```python
from build123d import *

# Parameters (mm, degrees)
F0_R     = 37.5
F1_DEPTH = 4
F2_R     = 37.5
F2_R_2   = 33.5
F3_DEPTH = 5
F4_R     = 35.6
F5_DEPTH = 5
F6_R     = 2.5
F7_DEPTH = 4.001
F8_R     = 5


with BuildPart() as f1:
    # F0 (on Top) → F1 (new body)
    with BuildSketch(Plane.XY):
        Circle(F0_R)
    extrude(amount=F1_DEPTH)

    # F2 (on face) → F3 (join)
    with BuildSketch(Plane.XY.offset(4)):
        Circle(F2_R)
        Circle(F2_R_2, mode=Mode.SUBTRACT)
    extrude(amount=F3_DEPTH)

    # F4 (on face) → F5 (cut)
    with BuildSketch(Plane.XY.offset(9)):
        Circle(F4_R)
    extrude(amount=-F5_DEPTH, mode=Mode.SUBTRACT)

    # F6 (on face) → F7 (cut, through all)
    with BuildSketch(Plane.XY.offset(4)):
        Circle(F6_R)
    extrude(amount=-F7_DEPTH, mode=Mode.SUBTRACT)

    # F8
    f8_edges = [f1.edges().sort_by_distance(p)[0] for p in [
        (-37.5, 0, 0),
    ]]
    fillet(f8_edges, radius=F8_R)


solid = f1.part
```
CAD build for the part. Positions are in the model's coordinates, mm. A direction names the side the tool comes from. Give positions to 0.01 mm unless a question says otherwise; leave off trailing zeros. Write each loop counter-clockwise with the first axis right and the second up, starting at its lowest first coordinate (ties: lowest second). Pieces come first, ordered by that corner, then holes. Notation, with made-up numbers: M 16,72 L 62,72 A18 cw 62,94 Z; hole C 37,16 d2. An arc over 180 degrees is marked long. Return JSON: item names as keys, results as strings. Group by question number.
(1) Flat gauge pins, fed straight in: pin 1 Ø5 at (x, y) = (15.5, -18.5) entering from +Z; pin 2 Ø6.5 at (x, y) = (0, 0) entering from -Z; pin 3 Ø3 at (x, z) = (-6, 5) entering from -Y; pin 4 Ø2 at (x, z) = (-5.5, 7) entering from +Y. Where does each tip first touch, or does it go through?
(2) Drill centre lines: L1, parallel to Y at x = 0, z = 7.7; L2, parallel to Z at x = 3.5, y = -16.5; L3, parallel to Y at x = 0, z = 2.5. Where is each one in solid material? Low to high. Write a range as [from, to].
(3) Band-saw the part on A-A (y = 0). Give the cut face in (x, z).
(4) 3-axis set-ups, long thin cutter, end or side, ignore diameter. For faces 4 (the face through (33, -14, 9)), 5 (the face through (0, -7, 4)): which of +Z, -Z, +X, -X, +Y, -Y reach the whole face in a straight line?
(5) Mould opens along X. For faces 1 (the face through (-4.88, 37.18, 6.97)), 2 (the face through (7, 0, 0)), 3 (the face through (-0.54, -2.44, 2.03)) say: pulls with the +X half, pulls with the -X half, needs draft (parallel to the pull), parting line crosses it, or undercut.
(6) Band-saw the part on C-C (z = 6.25). Give the cut face in (x, y), and give its area (3 significant figures).
(7) Band-saw the part on D-D (z = 1). Give the cut face in (x, y), and give its area (3 significant figures).
Entries:
{
 "1": {"pin 1": "stops at z = 4", "pin 2": "stops at z = 0", "pin 3": "stops at y = -37.23", "pin 4": "stops at y = 37.23"},
 "2": {"L1": "y = [-37.5, -35.6], [35.6, 37.5]", "L2": "z = [0, 4]", "L3": "y = [-36.83, -2.5], [2.5, 36.83]"},
 "3": {"outline": "M -37.5,5 A5 ccw -32.5,0 L -2.5,0 L -2.5,4 L -35.6,4 L -35.6,9 L -37.5,9 Z; M 2.5,0 L 32.5,0 A5 ccw 37.5,5 L 37.5,9 L 35.6,9 L 35.6,4 L 2.5,4 Z"},
 "4": {"face 4": "+Z, +X, -X, +Y, -Y", "face 5": "+Z"},
 "5": {"face 1": "parting line crosses it", "face 2": "needs draft", "face 3": "undercut"},
 "6": {"outline": "C 0,0 d75; hole C 0,0 d71.2", "area": "436 mm^2"},
 "7": {"outline": "C 0,0 d71; hole C 0,0 d5", "area": "3,940 mm^2"}
}
